Source: CAD feature listing. Evaluate the final solid. Frame: model axes, mm. Face numbers are marked on the shaded views. A direction names the side the tool comes from. Give positions to 0.01 mm unless a question says otherwise; leave off trailing zeros. Loops run counter-clockwise (first coordinate to the right, second up) from the corner with the lowest first, then second, coordinate; pieces in that order, holes last. Notation, with made-up numbers: M 25.5,85.5 L 57.5,85.5 A22 ccw 57.5,108.5 Z; hole C 41,18 d10. An arc over 180 degrees is marked long. Answer in a Markdown table with one row per item.
```python
from build123d import *

# Parameters (mm, degrees)
F1_DEPTH = 63.5
F0_W     = 15.748692
F0_H     = 4.7752
F2_DEPTH = 25.4
F3_DEPTH = 7.9375
F5_R     = 6.35


with BuildPart() as f1:
    # F0 (on Front) → F1 (new body, symmetric)
    with BuildSketch(Plane.XZ):
        Polygon((-41.275, 9.525), (-41.275, -9.525), (41.275, -9.525), (41.275, 9.525), (22.225, 9.525), align=None)
    extrude(amount=F1_DEPTH, both=True)

    # F0 (on Front) → F2 (join, symmetric)
    with BuildSketch(Plane.XZ):
        with Locations((68.199346, 40.4876)):
            Rectangle(F0_W, F0_H)
        with BuildLine():
            Line((22.225, 9.525), (41.275, 9.525))
            Line((41.275, 9.525), (41.275, 27.0002))
            ThreePointArc((41.275, 27.0002), (45.92468, 38.22552), (57.15, 42.8752))
            Line((57.15, 42.8752), (60.325, 42.8752))
            Line((60.325, 42.8752), (60.325, 61.9252))
            Line((60.325, 61.9252), (57.15, 61.9252))
            add(Edge.make_bspline(
                [(54.028564, 61.78543), (55.069144, 61.843048), (56.109775, 61.889675), (57.15, 61.9252)],
                knots=[108.777413, 108.777413, 108.777413, 108.777413, 111.504536, 111.504536, 111.504536, 111.504536], degree=3))
            ThreePointArc((54.028564, 61.78543), (31.374316, 50.566484), (22.225, 27.0002))
            Line((22.225, 27.0002), (22.225, 9.525))
        make_face()
    extrude(amount=F2_DEPTH, both=True)

    # F0 (on Front) → F3 (join, symmetric)
    with BuildSketch(Plane.XZ):
        with BuildLine():
            add(Edge.make_bspline(
                [(-41.275, 9.525), (-28.903485, 39.703747), (12.522665, 59.487237), (54.028564, 61.78543)],
                knots=[0, 0, 0, 0, 108.777413, 108.777413, 108.777413, 108.777413], degree=3))
            Line((-41.275, 9.525), (22.225, 9.525))
            Line((22.225, 9.525), (22.225, 27.0002))
            ThreePointArc((22.225, 27.0002), (31.374316, 50.566484), (54.028564, 61.78543))
        make_face()
    extrude(amount=F3_DEPTH, both=True)

    # F0 (on Front) → F4 (revolve)
    with BuildSketch(Plane.XZ):
        Polygon((76.073692, 66.675), (76.073692, 61.9252), (76.073692, 42.8752), (76.073692, 38.1), (111.125, 38.1), (111.125, 66.675), align=None)
    revolve(axis=Axis((76.073692, 0, 52.4002), (0, 0, 1)))

    # F5
    f5_edges = [f1.edges().sort_by_distance(p)[0] for p in [
        (41.275, -63.5, 0),
        (-41.275, -63.5, 0),
        (-41.275, 63.5, 0),
        (41.275, 63.5, 0),
    ]]
    fillet(f5_edges, radius=F5_R)


solid = f1.part
```
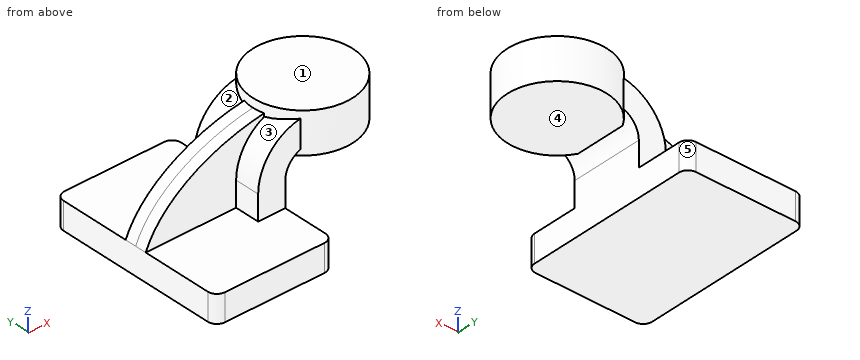
1) Section A-A, the plane y = -33. Return loops of the section in (x, z) (3 decimals).
Reply:
| item | result |
|---|---|
| outline | M -41.275,-9.525 L 41.275,-9.525 L 41.275,9.525 L -41.275,9.525 Z; M 64.259,38.1 L 87.889,38.1 L 87.889,66.675 L 64.259,66.675 Z |
2) Material intervals for L1, parallel to Y at x = 15, z = 21; L2, parallel to Z at x = 70, y = -8 (3 decimals); L3, parallel to X at y = -56, z = -6 (3 decimals), sorted ascending.
Reply:
| item | result |
|---|---|
| L1 | y = -7.94 to 7.94 |
| L2 | z = 38.1 to 66.675 |
| L3 | x = -41.275 to 41.275 |
3) Set-up query: the marked faces 1, 2, 3, 4 and 5. Return all of +Z, -Z, +X, -X, +Y, -Y with unobstructed straight access to the full face (end or side cutting, diameter ignored); none if empty.
Reply:
| item | result |
|---|---|
| face 1 | +Z, +X, -X, +Y, -Y |
| face 2 | +Z, -X, +Y |
| face 3 | +Z, -X, -Y |
| face 4 | -Z, +X, +Y, -Y |
| face 5 | +Z, -Z, +X, +Y |
4) Pin query (flat end, axial travel): pin 1 Ø15 at (x, z) = (35, 37.5) entering from -Y; pin 2 Ø6 at (y, z) = (15.5, 19) entering from +X (3 decimals); pin 3 Ø6 at (x, y) = (-20, 38.5) entering from +Z (3 decimals); pin 4 Ø4 at (x, y) = (46, 28.5) entering from -Z. Return the tip coordinate at first contact, or that it passes through.
Reply:
| item | result |
|---|---|
| pin 1 | stops at y = -25.4 |
| pin 2 | stops at x = 41.275 |
| pin 3 | stops at z = 9.525 |
| pin 4 | passes through |
5) Section B-B, the plane z = 2. Return loops of the section in (x, y) (3 decimals).
Reply:
| item | result |
|---|---|
| outline | M -41.275,-57.15 A6.35 ccw -34.925,-63.5 L 34.925,-63.5 A6.35 ccw 41.275,-57.15 L 41.275,57.15 A6.35 ccw 34.925,63.5 L -34.925,63.5 A6.35 ccw -41.275,57.15 Z |
6) Section C-C, the plane y = 42.5. Return loops of the section in (x, z) (3 decimals), then the cut area to 3 significant figures.
Reply:
| item | result |
|---|---|
| outline | M -41.275,-9.525 L 41.275,-9.525 L 41.275,9.525 L -41.275,9.525 Z |
| area | 1,570 mm² |
7) Section D-D, the plane x = 89.5. Return loops of the section in (y, z) (3 decimals), then the cut area to 3 significant figures.
Reply:
| item | result |
|---|---|
| outline | M -32.378,38.1 L 32.378,38.1 L 32.378,66.675 L -32.378,66.675 Z |
| area | 1,850 mm² |
